Input: part model. Units: mm. Frame: model coordinates. Face numbers are marked on the shaded views. A direction names the side the tool comes from. Round coordinates to 2 decimals unless told otherwise and drop trailing zeros. Loops run counter-clockwise (first coordinate to the right, second up) from the corner with the lowest first, then second, coordinate; pieces in that order, holes last.
1) Section B-B, the plane z = 26. Return loops of the section in (x, y), and give its area (3 significant figures).
2) First-contact query: pin 1 (6 mm diameter, centred on y = -6.5, z = 26, fed in from -X); pin 2 (5.5 mm diameter, centred on x = -1.5, z = 12, fed in from +Y); pin 3 (5 mm diameter, centred on x = 3.5, z = 16.5, fed in from +Y). Flat tips, straight axial feed; report the tip coordinate or a pass-through.
3) Section C-C, the plane x = 0. Return loops of the section in (y, z), and give its area (3 significant figures).
4) Access query for the marked faces 1 and 2. Directions: +Z, -Z, +X, -X, +Y, -Y. A direction counts if a zero-diameter tool reaches every point of the face in a straight line with its end or side. Return the directions, or none.
5) Ray query, line 1 along Z through (x, y) = (-3.75, -7); line 2 along Y through (x, z) = (-6.35, 26); line 3 along Y through (x, z) = (5.75, 26). Return the intervals inside material, ascending.
6) Draft query along Z for the marked faces 3, 4, 5 and 6. Return one class per face: pulls with the +Z half, pulls with the -Z half, needs draft (parallel to the pull), parting line crosses it, or undercut.
7) Section A-A, the plane y = 0. Return loops of the section in (x, z).
8) Section D-D, the plane y = 4.5. Return loops of the section in (x, z), and give its area (3 significant figures).
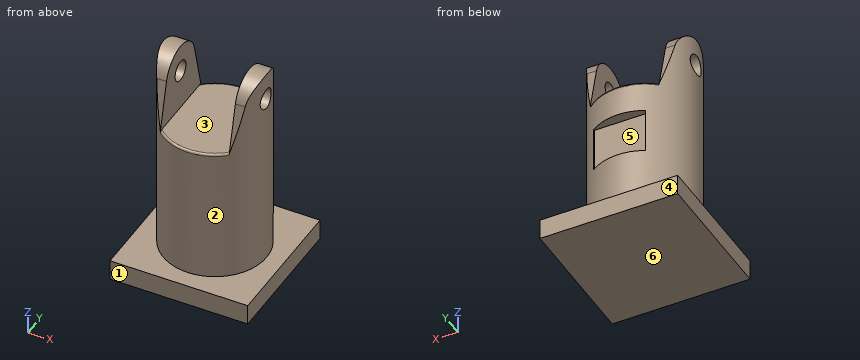
from build123d import *

# Parameters (mm, degrees)
CROQUIS1_R                 = 7.5
SALIENTE_EXTRUIR1_DEPTH    = 30
CORTAR_EXTRUIR1_DEPTH      = 32.819805153
CORTAR_EXTRUIR1_DEPTH_BACK = 10
CROQUIS2_W                 = 10
CROQUIS2_H                 = 15.47925891
CORTAR_EXTRUIR3_DEPTH      = 32.819805153
CORTAR_EXTRUIR3_DEPTH_BACK = 32.819805153
CORTAR_EXTRUIR4_DEPTH      = 32.819805295
CORTAR_EXTRUIR4_DEPTH_BACK = 32.819805295
CROQUIS4_R                 = 1.5
REDONDEO1_R                = 0.3
CROQUIS5_W                 = 20
CROQUIS5_H                 = 20
SALIENTE_EXTRUIR2_DEPTH    = 3
CORTAR_EXTRUIR5_START      = 6
CROQUIS6_W                 = 7.750181945
CROQUIS6_H                 = 6.56920184
CORTAR_EXTRUIR5_DEPTH      = 10


with BuildPart() as part:
    # Croquis1 → Saliente-Extruir1 (new body)
    with BuildSketch(Plane.XY):
        Circle(CROQUIS1_R)
    extrude(amount=SALIENTE_EXTRUIR1_DEPTH)

    # Croquis2 → Cortar-Extruir1 (cut, two sides: drawn at the far end of the back side and taken through both)
    with BuildSketch(Plane.XY.offset(30).offset(-CORTAR_EXTRUIR1_DEPTH_BACK)):
        Rectangle(CROQUIS2_W, CROQUIS2_H)
    extrude(amount=CORTAR_EXTRUIR1_DEPTH + CORTAR_EXTRUIR1_DEPTH_BACK, mode=Mode.SUBTRACT)

    # Croquis3 → Cortar-Extruir3 (cut, two sides: drawn at the far end of the back side and taken through both)
    with BuildSketch(Plane(origin=(0, 0, 0), x_dir=(0, 0, -1), z_dir=(1, 0, 0)).offset(-CORTAR_EXTRUIR3_DEPTH_BACK)):
        with BuildLine():
            Line((-20, 67.5), (-20, 7.5))
            Line((-20, 7.5), (-20, 5.590169944))
            Line((-20, 5.590169944), (-26.952923855, 3.884664175))
            ThreePointArc((-26.952923855, 3.884664175), (-29.999999999, -0.000262165), (-26.952744721, -3.885047998))
            Line((-26.952744721, -3.885047998), (-20, -5.590169944))
            Line((-20, -5.590169944), (-20, -7.5))
            Line((-20, -7.5), (-20, -67.5))
            Line((-20, -67.5), (-140, -67.5))
            Line((-140, -67.5), (-140, 67.5))
            Line((-140, 67.5), (-20, 67.5))
        make_face()
    extrude(amount=CORTAR_EXTRUIR3_DEPTH + CORTAR_EXTRUIR3_DEPTH_BACK, mode=Mode.SUBTRACT)

    # Croquis4 → Cortar-Extruir4 (cut, two sides: drawn at the far end of the back side and taken through both)
    with BuildSketch(Plane(origin=(0, 0, 0), x_dir=(0, 0, -1), z_dir=(1, 0, 0)).offset(-CORTAR_EXTRUIR4_DEPTH_BACK)):
        with Locations(Location((-26, -0.000169944, 0), (0, 0, 90))):
            Circle(CROQUIS4_R)
    extrude(amount=CORTAR_EXTRUIR4_DEPTH + CORTAR_EXTRUIR4_DEPTH_BACK, mode=Mode.SUBTRACT)

    # Redondeo1
    # the kernel refuses this fillet: 0.3 mm, written as the material it takes off along each edge
    with BuildSketch(Plane(origin=(0, 0, 20), x_dir=(0.7377709544179419, -0.6750511231138268, 0), z_dir=(0.6750511231138268, 0.7377709544179419, 0))) as redondeo1_piece_1_section:
        with BuildLine():
            CenterArc((7.5 - REDONDEO1_R, REDONDEO1_R), REDONDEO1_R, 270, 90)
            Line((7.5 - REDONDEO1_R, 0), (7.5, 0))
            Line((7.5, 0), (7.5, REDONDEO1_R))
        make_face()
    redondeo1_piece_1 = revolve(axis=Axis((0, 0, 20), (0, 0, -1)), revolution_arc=95.083759333, mode=Mode.PRIVATE)
    redondeo1_piece_1 = split(redondeo1_piece_1, bisect_by=Plane(origin=(5, -5.527382777, 19.949282133), z_dir=(-1, 0, 0)), keep=Keep.TOP, mode=Mode.PRIVATE)
    redondeo1_piece_1 = split(redondeo1_piece_1, bisect_by=Plane(origin=(-5, -5.527382777, 19.949282133), z_dir=(1, 0, 0)), keep=Keep.TOP, mode=Mode.PRIVATE)
    add(redondeo1_piece_1, mode=Mode.SUBTRACT)
    with BuildSketch(Plane(origin=(0, 0, 20), x_dir=(-0.737770954417942, 0.6750511231138266, 0), z_dir=(-0.6750511231138266, -0.737770954417942, 0))) as redondeo1_piece_2_section:
        with BuildLine():
            CenterArc((7.5 - REDONDEO1_R, REDONDEO1_R), REDONDEO1_R, 270, 90)
            Line((7.5 - REDONDEO1_R, 0), (7.5, 0))
            Line((7.5, 0), (7.5, REDONDEO1_R))
        make_face()
    redondeo1_piece_2 = revolve(axis=Axis((0, 0, 20), (0, 0, -1)), revolution_arc=95.083759333, mode=Mode.PRIVATE)
    redondeo1_piece_2 = split(redondeo1_piece_2, bisect_by=Plane(origin=(5, 5.527385531, 19.949280237), z_dir=(-1, 0, 0)), keep=Keep.TOP, mode=Mode.PRIVATE)
    redondeo1_piece_2 = split(redondeo1_piece_2, bisect_by=Plane(origin=(-5, 5.527385531, 19.949280237), z_dir=(1, 0, 0)), keep=Keep.TOP, mode=Mode.PRIVATE)
    add(redondeo1_piece_2, mode=Mode.SUBTRACT)

    # Croquis5 → Saliente-Extruir2 (add)
    with BuildSketch(Plane(origin=(0, 0, 0), x_dir=(-1, 0, 0), z_dir=(0, 0, -1))):
        Rectangle(CROQUIS5_W, CROQUIS5_H)
    extrude(amount=SALIENTE_EXTRUIR2_DEPTH)

    # Croquis6 → Cortar-Extruir5 (cut)
    with BuildSketch(Plane(origin=(0, 0, 0), x_dir=(1, 0, 0), z_dir=(0, 1, 0)).offset(CORTAR_EXTRUIR5_START)):
        with Locations((0.339668607, -12.101574185)):
            Rectangle(CROQUIS6_W, CROQUIS6_H)
    extrude(amount=CORTAR_EXTRUIR5_DEPTH, mode=Mode.SUBTRACT)


solid = part.part
Final values:
1. outline: (-7.35, -1.5) arc R7.5 ccw to (-6.27, -4.12) - (-5, -4.12) - (-5, -1.5) - close; (-7.35, 1.5) - (-5, 1.5) - (-5, 4.12) - (-6.27, 4.12) arc R7.5 ccw to start; (5, -4.12) - (6.27, -4.12) arc R7.5 ccw to (7.35, -1.5) - (5, -1.5) - close; (5, 1.5) - (7.35, 1.5) arc R7.5 ccw to (6.27, 4.12) - (5, 4.12) - close
1. area: 20.0 mm2
2. pin 1: stops at x = -6.63
2. pin 2: stops at y = 6.61
2. pin 3: stops at y = 7.43
3. outline: (-10, -3) - (10, -3) - (10, 0) - (7.5, 0) - (7.5, 8.82) - (6, 8.82) - (6, 15.39) - (7.5, 15.39) - (7.5, 19.7) arc R0.3 ccw to (7.2, 20) - (-7.2, 20) arc R0.3 ccw to (-7.5, 19.7) - (-7.5, 0) - (-10, 0) - close
3. area: 350 mm2
4. face 1: +Z, -Z, +X, -X, -Y
4. face 2: +Z
5. line 1: z = -3 to 0
5. line 2: y = -3.99 to -1.5, 1.5 to 3.99
5. line 3: y = -4.12 to -1.5, 1.5 to 4.12
6. face 3: pulls with the +Z half
6. face 4: needs draft
6. face 5: undercut
6. face 6: pulls with the -Z half
7. outline: (-10, -3) - (10, -3) - (10, 0) - (7.5, 0) - (7.5, 24.5) - (5, 24.5) - (5, 20) - (-5, 20) - (-5, 24.5) - (-7.5, 24.5) - (-7.5, 0) - (-10, 0) - close; (-7.5, 27.5) - (-5, 27.5) - (-5, 30) - (-7.5, 30) - close; (5, 27.5) - (7.5, 27.5) - (7.5, 30) - (5, 30) - close
8. outline: (-10, -3) - (10, -3) - (10, 0) - (6, 0) - (6, 24.44) - (5, 24.44) - (5, 20) - (-5, 20) - (-5, 24.44) - (-6, 24.44) - (-6, 0) - (-10, 0) - close
8. area: 309 mm2
